Can you work these out from the model? Positions are in its coordinate system, mm. A direction names the side the tool comes from. Coordinates: 2 decimals unless noted, no trailing zeros. Order: outer loops, then holes, each group sorted by start corner. A loop starts at its lowest first (then second) coordinate and runs counter-clockwise, first axis right, second up. Notation, with made-up numbers: (59, 0) -> (103, 0) arc R16 ccw to (103, 31) -> close; hole circle Ø9 at (19, 62.5). An arc over 180 degrees is marked (long way). Answer as a JSON object with one key per item and string values. Group by question number.
(1) If we mould it in two halves opening along X, with no side actions, what happens to faces 5 (the flat face through (29.609, 2.021, -29.787)), 6 (the flat face through (20, 1, 3)), 7 (the flat face through (-35, 2, 0))? For each: pulls with the +X half, pulls with the -X half, needs draft (parallel to the pull), parting line crosses it, or undercut.
(2) I want a section at A-A, the plane z = 11. List the corners of the cut face in (x, y) for me.
(3) For pin 1 (1 mm diameter, centred on x = -1, y = 1.5, fed in from +Z); pin 2 (0.6 mm diameter, centred on y = 0.5, z = -0.5, fed in from +X); pin 3 (3 mm diameter, centred on x = 19.5, z = -6, fed in from +Y); pin 4 (1.9 mm diameter, centred on x = -22.63, z = 31.11, fed in from +Y), each with a flat end and sliding along its axis, tell me the tip position at first contact or that it passes through.
(4) I want a section at D-D, the plane x = 13.5. List the corners of the cut face in (y, z) for me, plus the area to 3 significant figures.
(5) I need wall thicknesses on line 1 (X direction, y = 0.6, z = 0.5); line 2 (X direction, y = 2.3, z = 0); line 3 (Z direction, x = -7, y = 0.5). Which ranges of each line are inside material? Lowest first, please.
(6) I want a section at B-B, the plane z = 0. List the corners of the cut face in (x, y) for me.
(7) Which directions (+Z, -Z, +X, -X, +Y, -Y) give clear straight access to the entire face, cutting with the end or side of a thin tool? Please do faces 1 (the flat face through (-17.5, 1, -4)), 2 (the flat face through (29, 3, 0)), 3 (the flat face through (0, 2, -35)), 4 (the flat face through (17.99, 2.02, 35.54)).
(8) I want a section at C-C, the plane y = 3.15. State how many separate pieces and enclosed holes the cut face has, plus the area to 3 significant figures.
from build123d import *

# Parameters (mm, degrees)
SKETCH1_R           = 1.6
BOSS_EXTRUDE1_DEPTH = 4.1
CUT_EXTRUDE1_DEPTH  = 2
CUT_EXTRUDE2_DEPTH  = 52.043042311
SKETCH4_W           = 20
SKETCH4_H           = 35
CUT_EXTRUDE3_DEPTH  = 52.043042311


with BuildPart() as part:
    # Sketch1 → Boss-Extrude1 (new body)
    with BuildSketch(Plane(origin=(0, 0, 0), x_dir=(1, 0, 0), z_dir=(0, 1, 0))):
        Polygon((-35, 12.5), (-36.062322224, 23.334400163), (-23.334400163, 36.062322224), (-12.5, 35), (12.5, 35), (23.334400163, 36.062322224), (36.062322224, 23.334400163), (35, 12.5), (35, -12.5), (36.062322224, -23.334400163), (23.334400163, -36.062322224), (12.5, -35), (-12.5, -35), (-23.334400163, -36.062322224), (-36.062322224, -23.334400163), (-35, -12.5), align=None)
        with Locations(Location((22.627293382, 31.112574756, 0), (0, 0, 270))):
            Circle(SKETCH1_R, mode=Mode.SUBTRACT)
        with Locations(Location((31.112574756, 22.627293382, 0), (0, 0, 270))):
            Circle(SKETCH1_R, mode=Mode.SUBTRACT)
        with Locations(Location((31.112574756, -22.627293382, 0), (0, 0, 270))):
            Circle(SKETCH1_R, mode=Mode.SUBTRACT)
        with Locations(Location((22.627293382, -31.112574756, 0), (0, 0, 270))):
            Circle(SKETCH1_R, mode=Mode.SUBTRACT)
        with Locations(Location((-22.627293382, -31.112574756, 0), (0, 0, 270))):
            Circle(SKETCH1_R, mode=Mode.SUBTRACT)
        with Locations(Location((-31.112574756, -22.627293382, 0), (0, 0, 270))):
            Circle(SKETCH1_R, mode=Mode.SUBTRACT)
        with Locations(Location((-31.112574756, 22.627293382, 0), (0, 0, 270))):
            Circle(SKETCH1_R, mode=Mode.SUBTRACT)
        with Locations(Location((-22.627293382, 31.112574756, 0), (0, 0, 270))):
            Circle(SKETCH1_R, mode=Mode.SUBTRACT)
    extrude(amount=BOSS_EXTRUDE1_DEPTH)

    # Sketch2 → Cut-Extrude1 (cut)
    with BuildSketch(Plane(origin=(0, 4.1, 0), x_dir=(1, 0, 0), z_dir=(0, 1, 0))):
        Polygon((-17.668800325, 29), (17.668800325, 29), (29, 17.668800325), (29, -17.668800325), (17.668800325, -29), (-17.668800325, -29), (-29, -17.668800325), (-29, 17.668800325), align=None)
    extrude(amount=-CUT_EXTRUDE1_DEPTH, mode=Mode.SUBTRACT)

    # Sketch3 → Cut-Extrude2 (cut, through all)
    with BuildSketch(Plane(origin=(0, 2.1, 0), x_dir=(1, 0, 0), z_dir=(0, 1, 0))):
        with BuildLine():
            Line((-27.5, 6.7), (-27.5, -6.7))
            ThreePointArc((-27.5, -6.7), (-27.265685425, -7.265685425), (-26.7, -7.5))
            Line((-26.7, -7.5), (-18.3, -7.5))
            ThreePointArc((-18.3, -7.5), (-17.734314575, -7.265685425), (-17.5, -6.7))
            Line((-17.5, -6.7), (-17.5, -2.3))
            ThreePointArc((-17.5, -2.3), (-17.734314575, -1.734314575), (-18.3, -1.5))
            Line((-18.3, -1.5), (-19.2, -1.5))
            ThreePointArc((-19.2, -1.5), (-19.765685425, -1.734314575), (-20, -2.3))
            Line((-20, -2.3), (-20, -4.2))
            ThreePointArc((-20, -4.2), (-20.234314575, -4.765685425), (-20.8, -5))
            Line((-20.8, -5), (-24.02, -5))
            ThreePointArc((-24.02, -5), (-24.585685425, -4.765685425), (-24.82, -4.2))
            Line((-24.82, -4.2), (-24.82, 4.22))
            ThreePointArc((-24.82, 4.22), (-24.585685425, 4.785685425), (-24.02, 5.02))
            Line((-24.02, 5.02), (-20.8, 5.02))
            ThreePointArc((-20.8, 5.02), (-20.234314575, 4.785685425), (-20, 4.22))
            Line((-20, 4.22), (-20, 2.3))
            ThreePointArc((-20, 2.3), (-19.765685425, 1.734314575), (-19.2, 1.5))
            Line((-19.2, 1.5), (-18.3, 1.5))
            ThreePointArc((-18.3, 1.5), (-17.734314575, 1.734314575), (-17.5, 2.3))
            Line((-17.5, 2.3), (-17.5, 6.7))
            ThreePointArc((-17.5, 6.7), (-17.734314575, 7.265685425), (-18.3, 7.5))
            Line((-18.3, 7.5), (-26.7, 7.5))
            ThreePointArc((-26.7, 7.5), (-27.265685425, 7.265685425), (-27.5, 6.7))
        make_face()
        with BuildLine():
            Line((18.3, 7.5), (26.7, 7.5))
            ThreePointArc((26.7, 7.5), (27.265685425, 7.265685425), (27.5, 6.7))
            Line((27.5, 6.7), (27.5, -6.7))
            ThreePointArc((27.5, -6.7), (27.265685425, -7.265685425), (26.7, -7.5))
            Line((26.7, -7.5), (18.3, -7.5))
            ThreePointArc((18.3, -7.5), (17.734314575, -7.265685425), (17.5, -6.7))
            Line((17.5, -6.7), (17.5, -2.3))
            ThreePointArc((17.5, -2.3), (17.734314575, -1.734314575), (18.3, -1.5))
            Line((18.3, -1.5), (19.2, -1.5))
            ThreePointArc((19.2, -1.5), (19.765685425, -1.734314575), (20, -2.3))
            Line((20, -2.3), (20, -4.2))
            ThreePointArc((20, -4.2), (20.234314575, -4.765685425), (20.8, -5))
            Line((20.8, -5), (24.02, -5))
            ThreePointArc((24.02, -5), (24.585685425, -4.765685425), (24.82, -4.2))
            Line((24.82, -4.2), (24.82, 4.22))
            ThreePointArc((24.82, 4.22), (24.585685425, 4.785685425), (24.02, 5.02))
            Line((24.02, 5.02), (20.8, 5.02))
            ThreePointArc((20.8, 5.02), (20.234314575, 4.785685425), (20, 4.22))
            Line((20, 4.22), (20, 2.3))
            ThreePointArc((20, 2.3), (19.765685425, 1.734314575), (19.2, 1.5))
            Line((19.2, 1.5), (18.3, 1.5))
            ThreePointArc((18.3, 1.5), (17.734314575, 1.734314575), (17.5, 2.3))
            Line((17.5, 2.3), (17.5, 6.7))
            ThreePointArc((17.5, 6.7), (17.734314575, 7.265685425), (18.3, 7.5))
        make_face()
    extrude(amount=-CUT_EXTRUDE2_DEPTH, mode=Mode.SUBTRACT)

    # Sketch4 → Cut-Extrude3 (cut, through all)
    with BuildSketch(Plane(origin=(0, 2.1, 0), x_dir=(1, 0, 0), z_dir=(0, 1, 0))):
        Rectangle(SKETCH4_W, SKETCH4_H)
    extrude(amount=-CUT_EXTRUDE3_DEPTH, mode=Mode.SUBTRACT)


solid = part.part
Computed values:
{
 "1": {"face 5": "pulls with the +X half", "face 6": "undercut", "face 7": "pulls with the -X half"},
 "2": {"outline": "(-35, 0) -> (-10, 0) -> (-10, 2.1) -> (-29, 2.1) -> (-29, 4.1) -> (-35, 4.1) -> close; (10, 0) -> (35, 0) -> (35, 4.1) -> (29, 4.1) -> (29, 2.1) -> (10, 2.1) -> close"},
 "3": {"pin 1": "stops at z = 35", "pin 2": "stops at x = 35", "pin 3": "stops at y = 2.1", "pin 4": "passes through"},
 "4": {"outline": "(0, -35.1) -> (4.1, -35.1) -> (4.1, -29) -> (2.1, -29) -> (2.1, 29) -> (4.1, 29) -> (4.1, 35.1) -> (0, 35.1) -> close", "area": "172 mm2"},
 "5": {"line 1": "x = -35 to -27.5, -24.82 to -10, 10 to 24.82, 27.5 to 35", "line 2": "x = -35 to -29, 29 to 35", "line 3": "z = -35 to -17.5, 17.5 to 35"},
 "6": {"outline": "(-35, 0) -> (-27.5, 0) -> (-27.5, 2.1) -> (-29, 2.1) -> (-29, 4.1) -> (-35, 4.1) -> close; (-24.82, 0) -> (-10, 0) -> (-10, 2.1) -> (-24.82, 2.1) -> close; (10, 0) -> (24.82, 0) -> (24.82, 2.1) -> (10, 2.1) -> close; (27.5, 0) -> (35, 0) -> (35, 4.1) -> (29, 4.1) -> (29, 2.1) -> (27.5, 2.1) -> close"},
 "7": {"face 1": "+Y, -Y", "face 2": "+Y", "face 3": "-Z, +Y, -Y", "face 4": "+Z, +Y, -Y"},
 "8": {"separate pieces": "1", "enclosed holes": "9", "area": "1,550 mm2"}
}
